Verification items for the finished model (mm, model axes). Face numbers are marked on the shaded views. A direction names the side the tool comes from. Coordinates: 2 decimals unless noted, no trailing zeros. Order: outer loops, then holes, each group sorted by start corner. A loop starts at its lowest first (then second) coordinate and runs counter-clockwise, first axis right, second up. Notation, with made-up numbers: M 68.25,7.5 L 92.25,7.5 A31 cw 92.25,37.5 Z; hole C 71.25,52.5 d10. An arc over 180 degrees is marked long. Answer as a JSON object with one key per item and string values. Group by question number.
(1) Cross-section at B-B (y = 20). Enter the section's corners in (x, z), plus the area to 3 significant figures.
(2) Cross-section at D-D (y = 14.25). Enter the section's corners in (x, z), plus the area to 3 significant figures.
(3) Material ranges on line 1 (Z direction, x = 9, y = 15.25); line 2 (Z direction, x = 11.15, y = 20), recorded low to high.
(4) Mould release check, pull along Z, two halves, no side actions. Record for the marked faces 6, 7 and 8: released by +Z, released by -Z, zero draft, split by the parting line, or undercut.
(5) Cross-section at A-A (x = 10.75). Enter the section's corners in (y, z), plus the area to 3 significant figures.
(6) Cross-section at C-C (z = 22.5). Enter the section's corners in (x, y), plus the area to 3 significant figures.
(7) Access from +Z, -Z, +X, -X, +Y, -Y to the whole of each face (thin tool, end or side, straight path). Record for the marked faces 1, 2, 3, 4 and 5.
(8) Gauge pin test, flat ends, axial feed: pin 1 Ø0.8 at (x, z) = (-0.5, 20) entering from +Y; pin 2 Ø1.8 at (x, z) = (9.5, 36) entering from -Y; pin 3 Ø10 at (y, z) = (20, 22.5) entering from +X. Record the tip position at first contact, or that the pin passes through.
from build123d import *

# Parameters (mm, degrees)
CYLINDER005_R      = 3.15
CYLINDER005_DEPTH  = 18
CYLINDER004_R      = 6.5
CYLINDER004_DEPTH  = 18
BOX011_W           = 15
BOX011_H           = 7.75
BOX011_DEPTH       = 35.5
BOX009_W           = 15
BOX009_H           = 20
BOX009_DEPTH       = 45
BOX010_W           = 15
BOX010_H           = 7.75
BOX010_DEPTH       = 23.5
CHAMFER003012_SIZE = 0.4
CHAMFER003013_SIZE = 1
CHAMFER003014_SIZE = 3
BOX012_W           = 10
BOX012_H           = 7.8
BOX012_DEPTH       = 4.75
BOX013_W           = 10
BOX013_H           = 7.8
BOX013_DEPTH       = 4.75
BOX014_W           = 10
BOX014_H           = 7.8
BOX014_DEPTH       = 23.5
CHAMFER003008_SIZE = 1


with BuildPart() as cylinder005:
    # Cylinder005 → Cylinder005 (new body)
    with BuildSketch(Plane(origin=(-3.5, 20, 22.5), x_dir=(0, 0, -1), z_dir=(1, 0, 0))):
        Circle(CYLINDER005_R)
    extrude(amount=CYLINDER005_DEPTH)


with BuildPart() as cylinder004:
    # Cylinder004 → Cylinder004 (new body)
    with BuildSketch(Plane(origin=(10, 20, 22.5), x_dir=(0, 0, -1), z_dir=(1, 0, 0))):
        Circle(CYLINDER004_R)
    extrude(amount=CYLINDER004_DEPTH)


with BuildPart() as cube011:
    # Box011 → Box011 (new body)
    with BuildSketch(Plane(origin=(0, 10, 4.75), x_dir=(1, 0, 0), z_dir=(0, 0, 1))):
        with Locations((7.5, 3.875)):
            Rectangle(BOX011_W, BOX011_H)
    extrude(amount=BOX011_DEPTH)


with BuildPart() as cut008004003004014002002005003002:
    # Box009 → Box009 (new body)
    with BuildSketch(Plane(origin=(0, 10, 0), x_dir=(1, 0, 0), z_dir=(0, 0, 1))):
        with Locations((7.5, 10)):
            Rectangle(BOX009_W, BOX009_H)
    extrude(amount=BOX009_DEPTH)

    # Cut008004003004014002002005003002: cut Cube011
    add(cube011.part, mode=Mode.SUBTRACT)


with BuildPart() as chamfer003014:
    # Box010 → Box010 (new body)
    with BuildSketch(Plane(origin=(0, 11.75, 10.75), x_dir=(1, 0, 0), z_dir=(0, 0, 1))):
        with Locations((7.5, 3.875)):
            Rectangle(BOX010_W, BOX010_H)
    extrude(amount=BOX010_DEPTH)

    # Fusion008: union Cut008004003004014002002005003002
    add(cut008004003004014002002005003002.part)

    # Chamfer003012
    chamfer003012_edges = [chamfer003014.edges().sort_by_distance(p)[0] for p in [
        (7.5, 10, 40.25),
        (7.5, 10, 4.75),
        (7.5, 10, 0),
        (7.5, 10, 45),
    ]]
    chamfer(chamfer003012_edges, length=CHAMFER003012_SIZE)

    # Chamfer003013
    chamfer003013_edges = [chamfer003014.edges().sort_by_distance(p)[0] for p in [
        (7.5, 11.75, 10.75),
        (7.5, 11.75, 34.25),
    ]]
    chamfer(chamfer003013_edges, length=CHAMFER003013_SIZE)

    # Chamfer003014
    chamfer003014_edges = [chamfer003014.edges().sort_by_distance(p)[0] for p in [
        (7.5, 30, 0),
        (7.5, 30, 45),
    ]]
    chamfer(chamfer003014_edges, length=CHAMFER003014_SIZE)


with BuildPart() as cube012:
    # Box012 → Box012 (new body)
    with BuildSketch(Plane(origin=(-1, 16.1, 0), x_dir=(1, 0, 0), z_dir=(0, 0, 1))):
        with Locations((5, 3.9)):
            Rectangle(BOX012_W, BOX012_H)
    extrude(amount=BOX012_DEPTH)


with BuildPart() as cube013:
    # Box013 → Box013 (new body)
    with BuildSketch(Plane(origin=(-1, 16.1, 40.25), x_dir=(1, 0, 0), z_dir=(0, 0, 1))):
        with Locations((5, 3.9)):
            Rectangle(BOX013_W, BOX013_H)
    extrude(amount=BOX013_DEPTH)


with BuildPart() as din_stopper:
    # Box014 → Box014 (new body)
    with BuildSketch(Plane(origin=(-1, 16.1, 10.75), x_dir=(1, 0, 0), z_dir=(0, 0, 1))):
        with Locations((5, 3.9)):
            Rectangle(BOX014_W, BOX014_H)
    extrude(amount=BOX014_DEPTH)

    # Fusion005: union Cube012, Cube013
    add(cube012.part)
    add(cube013.part)

    # Chamfer003008
    chamfer003008_edges = [din_stopper.edges().sort_by_distance(p)[0] for p in [
        (-1, 20, 34.25),
        (-1, 20, 10.75),
        (-1, 20, 4.75),
        (-1, 20, 0),
        (-1, 20, 45),
        (-1, 20, 40.25),
    ]]
    chamfer(chamfer003008_edges, length=CHAMFER003008_SIZE)

    # Fusion009: union Chamfer003014
    add(chamfer003014.part)

    # Cut008004003004014002002005003003: cut Cylinder004
    add(cylinder004.part, mode=Mode.SUBTRACT)

    # Cut008004003004014002002005003004: cut Cylinder005
    add(cylinder005.part, mode=Mode.SUBTRACT)


solid = din_stopper.part
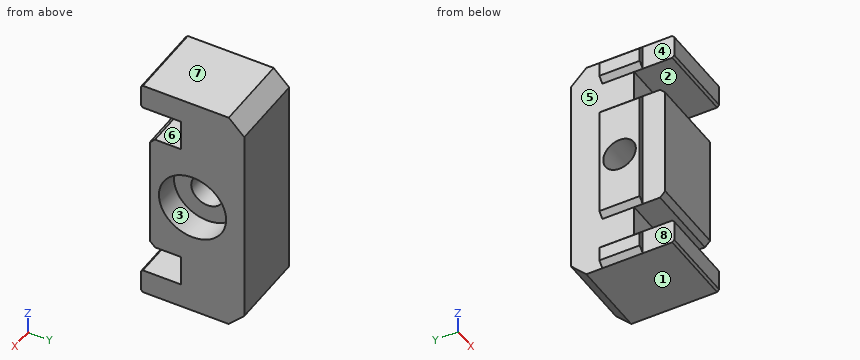
Taken from the geometry:
{
 "1": {"outline": "M -1,1 L 0,0 L 15,0 L 15,16 L 10,16 L 10,19.35 L -1,19.35 L -1,11.75 L 0,10.75 L 0,4.75 L -1,3.75 Z; M -1,25.65 L 10,25.65 L 10,29 L 15,29 L 15,45 L 0,45 L -1,44 L -1,41.25 L 0,40.25 L 0,34.25 L -1,33.25 Z", "area": "571 mm²"},
 "2": {"outline": "M 0,0 L 15,0 L 15,4.75 L 0,4.75 Z; M 0,10.75 L 15,10.75 L 15,19.47 L 10,19.47 L 10,25.53 L 15,25.53 L 15,34.25 L 0,34.25 Z; M 0,40.25 L 15,40.25 L 15,45 L 0,45 Z", "area": "465 mm²"},
 "3": {"line 1": "z = 0 to 4.75, 10.75 to 34.25, 40.25 to 45", "line 2": "z = 0 to 16, 29 to 45"},
 "4": {"face 6": "undercut", "face 7": "released by +Z", "face 8": "zero draft"},
 "5": {"outline": "M 10,0.4 L 10.4,0 L 27,0 L 30,3 L 30,42 L 27,45 L 10.4,45 L 10,44.6 L 10,40.65 L 10.4,40.25 L 17.75,40.25 L 17.75,34.25 L 12.75,34.25 L 11.75,33.25 L 11.75,11.75 L 12.75,10.75 L 17.75,10.75 L 17.75,4.75 L 10.4,4.75 L 10,4.35 Z; hole C 20,22.5 d13", "area": "623 mm²"},
 "6": {"outline": "M -1,16.1 L 0,16.1 L 0,11.75 L 15,11.75 L 15,13.5 L 10,13.5 L 10,16.85 L -1,16.85 Z; M -1,23.15 L 10,23.15 L 10,26.5 L 15,26.5 L 15,30 L 0,30 L 0,23.9 L -1,23.9 Z", "area": "147 mm²"},
 "7": {"face 1": "-Z, +X, -X, +Y, -Y", "face 2": "+X, -X, -Y", "face 3": "+X", "face 4": "+Z, -Z, -X, -Y", "face 5": "-X, +Y"},
 "8": {"pin 1": "stops at y = 23.9", "pin 2": "stops at y = 17.75", "pin 3": "stops at x = 10"}
}
